The listing builds one solid part. Answer for the finished solid, in the listing's coordinates (mm). Face numbers are marked on the shaded views. A direction names the side the tool comes from. Coordinates: 2 decimals unless noted, no trailing zeros. Loops run counter-clockwise (first coordinate to the right, second up) from the corner with the lowest first, then second, coordinate; pieces in that order, holes last. Notation, with made-up numbers: M 51.5,56 L 95.5,56 A28 cw 95.5,90 Z; hole C 54.25,27 d1. An arc over 180 degrees is marked long. Answer as a JSON object with one key per item and string values. Group by question number.
1. A cutting plane is placed at A-A on z = 28.5. Give the vertices of the cut face in (x, y), and give its area (3 significant figures).
2. Straight lines are drawn through the part: L1, parallel to X at y = 38, z = 184.5; L2, parallel to Y at x = -83, z = 159.5; L3, parallel to Z at x = -156, y = 5. For each, find the intervals that lie inside material, in ascending order.
3. For the marked faces 4 and 5, determine the directions among +Z, -Z, +X, -X, +Y, -Y from which every point of the face is accessible in a straight line to the end or side of a thin tool.
4. Determine the mould class of the marked faces 1, 2 and 3 for opening direction X: released by +X, released by -X, zero draft, split by the parting line, or undercut.
5. Given pin 1 (3 mm diameter, centred on y = 23.6, z = 189.53, fed in from +X); pin 2 (0.9 mm diameter, centred on x = -253, y = 20.5, fed in from -Z); pin 3 (1.4 mm diameter, centred on y = 42, z = 236.5, fed in from -X); pin 4 (1.8 mm diameter, centred on y = 0, z = 235, fed in from -X), each flat-ended and moving along its own axis, determine where each tip first touches the part or whether it passes through.
6. A cutting plane is placed at C-C on x = -100. Give the vertices of the cut face in (y, z).
7. A cutting plane is placed at B-B on z = 90. Give the vertices of the cut face in (x, y).
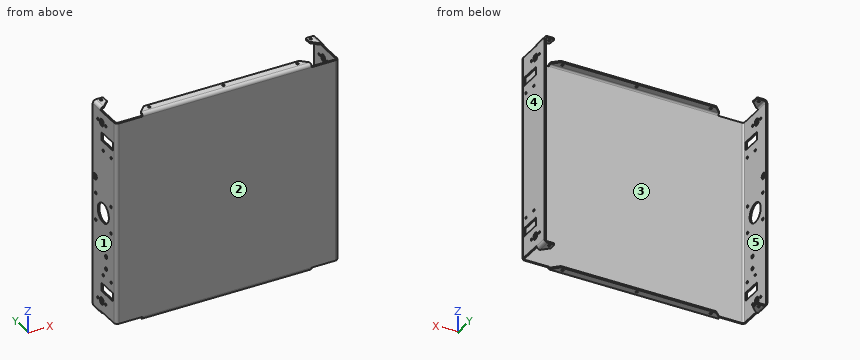
from build123d import *

# Parameters (mm, degrees)
F1_DEPTH  = 233.737836
F2_W      = 1.70942
F2_H      = 15.875
F2_W_2    = 194.007206
F2_H_2    = 1.70942
F3_DEPTH  = 3.69316
F4_W      = 1.70942
F4_H      = 15.875
F4_W_2    = 194.007206
F4_H_2    = 1.70942
F5_DEPTH  = 3.69316
F6_W      = 194.007206
F6_H      = 1.70942
F7_DEPTH  = 9.92124
F8_W      = 15.875
F8_H      = 1.70942
F9_DEPTH  = 9.92124
F10_W     = 15.875
F10_H     = 1.70942
F11_DEPTH = 9.92124
F12_R     = 1.98374
F13_R     = 3.69316
F14_SIZE  = 7.9375
F15_R     = 1.35255
F16_DEPTH = 241.124156
F17_R     = 1.35255
F17_R_2   = 4
F17_W     = 24
F17_H     = 9.532924
F17_H_2   = 9.532925
F18_DEPTH = 255.655496
F19_R     = 0.762
F20_R     = 11.253
F20_R_2   = 1.5
F20_R_3   = 3.5
F20_R_4   = 2.15265
F21_DEPTH = 1.70942


with BuildPart() as f1:
    # F0 (on Top) → F1 (new body)
    with BuildSketch(Plane.XY):
        Polygon((0, 44.989725), (0, 0), (-252.236656, 0), (-252.236656, 44.989725), (-253.946076, 44.989725), (-253.946076, -1.70942), (1.70942, -1.70942), (1.70942, 44.989725), align=None)
    extrude(amount=F1_DEPTH)

    # F2 (on face) → F3 (join)
    with BuildSketch(Plane(origin=(0, 0, 0), x_dir=(1, 0, 0), z_dir=(0, 0, -1))):
        with Locations((0.85471, -37.052225)):
            Rectangle(F2_W, F2_H)
        with Locations((-126.118328, 0.85471)):
            Rectangle(F2_W_2, F2_H_2)
        with Locations((-253.091366, -37.052225)):
            Rectangle(F2_W, F2_H)
    extrude(amount=F3_DEPTH)

    # F4 (on face) → F5 (join)
    with BuildSketch(Plane.XY.offset(233.737836)):
        with Locations((-253.091366, 37.052225)):
            Rectangle(F4_W, F4_H)
        with Locations((0.85471, 37.052225)):
            Rectangle(F4_W, F4_H)
        with Locations((-126.118328, -0.85471)):
            Rectangle(F4_W_2, F4_H_2)
    extrude(amount=F5_DEPTH)

    # F6 (on face) → F7 (join)
    with BuildSketch(Plane(origin=(0, 0, 0), x_dir=(-1, 0, 0), z_dir=(0, 1, 0))):
        with Locations((126.118328, -2.83845)):
            Rectangle(F6_W, F6_H)
        with Locations((126.118328, 236.576286)):
            Rectangle(F6_W, F6_H)
    extrude(amount=F7_DEPTH)

    # F8 (on face) → F9 (join)
    with BuildSketch(Plane.YZ.offset(-252.236656)):
        with Locations((37.052225, 236.576286)):
            Rectangle(F8_W, F8_H)
        with Locations((37.052225, -2.83845)):
            Rectangle(F8_W, F8_H)
    extrude(amount=F9_DEPTH)

    # F10 (on face) → F11 (join)
    with BuildSketch(Plane(origin=(0, 0, 0), x_dir=(0, -1, 0), z_dir=(-1, 0, 0))):
        with Locations((-37.052225, -2.83845)):
            Rectangle(F10_W, F10_H)
        with Locations((-37.052225, 236.576286)):
            Rectangle(F10_W, F10_H)
    extrude(amount=F11_DEPTH)

    # F12
    f12_edges = [f1.edges().sort_by_distance(p)[0] for p in [
        (0, 37.052225, 235.721576),
        (-126.118328, 0, 235.721576),
        (-252.236656, 37.052225, 235.721576),
        (-252.236656, 37.052225, -1.98374),
        (-126.118328, 0, -1.98374),
        (0, 37.052225, -1.98374),
        (0, 0, 116.868918),
        (-252.236656, 0, 116.868918),
    ]]
    fillet(f12_edges, radius=F12_R)

    # F13
    f13_edges = [f1.edges().sort_by_distance(p)[0] for p in [
        (-253.946076, 37.052225, -3.69316),
        (-126.118328, -1.70942, -3.69316),
        (-253.946076, -1.70942, 116.868918),
        (-126.118328, -1.70942, 237.430996),
        (-253.946076, 37.052225, 237.430996),
        (1.70942, 37.052225, -3.69316),
        (1.70942, -1.70942, 116.868918),
        (1.70942, 37.052225, 237.430996),
    ]]
    fillet(f13_edges, radius=F13_R)

    # F14
    f14_edges = [f1.edges().sort_by_distance(p)[0] for p in [
        (-242.315416, 29.114725, 236.576286),
        (-223.121931, 9.92124, 236.576286),
        (-29.114725, 9.92124, 236.576286),
        (-9.92124, 29.114725, 236.576286),
        (-29.114725, 9.92124, -2.83845),
        (-9.92124, 29.114725, -2.83845),
        (-242.315416, 29.114725, -2.83845),
        (-223.121931, 9.92124, -2.83845),
    ]]
    chamfer(f14_edges, length=F14_SIZE)

    # F15 (on face) → F16 (cut, through all)
    with BuildSketch(Plane(origin=(0, 0, -3.69316), x_dir=(1, 0, 0), z_dir=(0, 0, -1))):
        with Locations((-41.020975, -5.95249)):
            Circle(F15_R)
        with Locations((-126.118328, -5.95249)):
            Circle(F15_R)
        with Locations((-211.215681, -5.95249)):
            Circle(F15_R)
        with Locations((-246.284166, -41.020975)):
            Circle(F15_R)
        with Locations((-5.95249, -41.020975)):
            Circle(F15_R)
    extrude(amount=-F16_DEPTH, mode=Mode.SUBTRACT)

    # F17 (on face) → F18 (cut, through all)
    with BuildSketch(Plane(origin=(-253.946076, 0, 0), x_dir=(0, -1, 0), z_dir=(-1, 0, 0))):
        with Locations((-34.594617, 12.78067)):
            Circle(F17_R)
        with Locations((-18.657117, 12.78067)):
            Circle(F17_R)
        with Locations((-18.657117, 220.957165)):
            Circle(F17_R)
        with Locations((-34.594617, 220.957165)):
            Circle(F17_R)
        with Locations((-26.625867, 220.957165)):
            Circle(F17_R_2)
        with Locations((-26.625867, 12.78067)):
            Circle(F17_R_2)
        with Locations((-15.57124, 204.694663)):
            Rectangle(F17_W, F17_H)
        with Locations((-15.57124, 29.043172)):
            Rectangle(F17_W, F17_H_2)
        with Locations((-23.60249, 44.205093)):
            Circle(F17_R)
        with Locations((-7.53999, 44.205093)):
            Circle(F17_R)
        with Locations((-23.60249, 189.532743)):
            Circle(F17_R)
        with Locations((-7.53999, 189.532743)):
            Circle(F17_R)
    extrude(amount=-F18_DEPTH, mode=Mode.SUBTRACT)

    # F19
    f19_edges = [f1.edges().sort_by_distance(p)[0] for p in [
        (-242.315416, 44.989725, -2.83845),
        (-242.315416, 44.989725, 236.576286),
        (-9.92124, 44.989725, 236.576286),
        (-9.92124, 44.989725, -2.83845),
    ]]
    fillet(f19_edges, radius=F19_R)

    # F20 (on face) → F21 (cut, through all)
    with BuildSketch(Plane(origin=(-253.946076, 0, 0), x_dir=(0, -1, 0), z_dir=(-1, 0, 0))):
        with Locations((-23.486732, 116.868918)):
            Circle(F20_R)
        with Locations((-38.986727, 132.368912)):
            Circle(F20_R_2)
        with Locations((-7.986738, 132.368912)):
            Circle(F20_R_2)
        with Locations((-7.986738, 101.368924)):
            Circle(F20_R_2)
        with Locations((-38.986727, 101.368924)):
            Circle(F20_R_2)
        with Locations((-40.239725, 151.07191)):
            Circle(F20_R_3)
        with Locations((-17.840581, 68.833657)):
            Circle(F20_R_4)
        with Locations((-17.840581, 54.546157)):
            Circle(F20_R_4)
    extrude(amount=-F21_DEPTH, mode=Mode.SUBTRACT)


solid = f1.part
From the geometry:
{
 "1": {"outline": "M -253.95,1.98 A3.69 ccw -250.25,-1.71 L -1.98,-1.71 A3.69 ccw 1.71,1.98 L 1.71,3.57 L 0,3.57 L 0,1.98 A1.98 cw -1.98,0 L -250.25,0 A1.98 cw -252.24,1.98 L -252.24,3.57 L -253.95,3.57 Z; M -253.95,27.57 L -252.24,27.57 L -252.24,44.99 L -253.95,44.99 Z; M 0,27.57 L 1.71,27.57 L 1.71,44.99 L 0,44.99 Z", "area": "505 mm²"},
 "2": {"L1": "x = -253.95 to -252.24, 0 to 1.71", "L2": "y = -1.71 to 0", "L3": "z = -3.69 to -1.98, 235.72 to 237.43"},
 "3": {"face 4": "+Z, -Z, +X, +Y, -Y", "face 5": "+Y"},
 "4": {"face 1": "released by -X", "face 2": "zero draft", "face 3": "undercut"},
 "5": {"pin 1": "stops at x = 1.71", "pin 2": "stops at z = 0", "pin 3": "stops at x = -253.32", "pin 4": "stops at x = -223.12"},
 "6": {"outline": "M -1.71,0 A3.69 ccw 1.98,-3.69 L 9.92,-3.69 L 9.92,-1.98 L 1.98,-1.98 A1.98 cw 0,0 L 0,233.74 A1.98 cw 1.98,235.72 L 9.92,235.72 L 9.92,237.43 L 1.98,237.43 A3.69 ccw -1.71,233.74 Z"},
 "7": {"outline": "M -253.95,1.98 A3.69 ccw -250.25,-1.71 L -1.98,-1.71 A3.69 ccw 1.71,1.98 L 1.71,44.99 L 0,44.99 L 0,1.98 A1.98 cw -1.98,0 L -250.25,0 A1.98 cw -252.24,1.98 L -252.24,44.99 L -253.95,44.99 Z"}
}
